Verification items for the finished model (mm, model axes). Give positions to 0.01 mm unless a question says otherwise; leave off trailing zeros. Order: outer loops, then holes, each group sorted by start corner. A loop starts at its lowest first (then second) coordinate and runs counter-clockwise, first axis right, second up.
from build123d import *

# Parameters (mm, degrees)
BOSS_EXTRUDE2_DEPTH     = 3
CUT_EXTRUDE1_DEPTH      = 330.393231219
CUT_EXTRUDE1_DEPTH_BACK = 3
SKETCH4_W               = 17.5
SKETCH4_H               = 12
CUT_EXTRUDE2_DEPTH      = 10
SKETCH5_R               = 5.7
CUT_EXTRUDE3_DEPTH      = 10
SKETCH6_R               = 6.5
CUT_EXTRUDE4_DEPTH      = 10
SKETCH7_R               = 1.5
CUT_EXTRUDE5_DEPTH      = 10


with BuildPart() as part:
    # Sketch1 → Boss-Extrude2 (new body)
    with BuildSketch(Plane(origin=(0, 0, 0), x_dir=(0, 0, -1), z_dir=(1, 0, 0))):
        Polygon((18.855403516, 70), (318.855403516, 70), (318.855403516, 55), (321.855403516, 55), (321.855403516, 15), (318.855403516, 15), (318.855403516, 0), (18.855403516, 0), (18.855403516, 15), (15.855403516, 15), (15.855403516, 55), (18.855403516, 55), align=None)
    extrude(amount=BOSS_EXTRUDE2_DEPTH)

    # Sketch3 → Cut-Extrude1 (cut, two sides: drawn at the far end of the back side and taken through both)
    with BuildSketch(Plane(origin=(3, 0, 0), x_dir=(0, 0, -1), z_dir=(1, 0, 0)).offset(-CUT_EXTRUDE1_DEPTH_BACK)):
        Polygon((48.855403516, 643.663019898), (48.855403516, 70), (48.855403516, 67), (288.855403516, 67), (288.855403516, 70), (288.855403516, 643.663019898), (288.855403516, 1790.989059693), (48.855403516, 1790.989059693), align=None)
    extrude(amount=CUT_EXTRUDE1_DEPTH + CUT_EXTRUDE1_DEPTH_BACK, mode=Mode.SUBTRACT)

    # Sketch4 → Cut-Extrude2 (cut)
    with BuildSketch(Plane(origin=(3, 0, 0), x_dir=(0, 0, -1), z_dir=(1, 0, 0))):
        with Locations((250.105403516, 31)):
            Rectangle(SKETCH4_W, SKETCH4_H)
    extrude(amount=-CUT_EXTRUDE2_DEPTH, mode=Mode.SUBTRACT)

    # Sketch5 → Cut-Extrude3 (cut)
    with BuildSketch(Plane(origin=(3, 0, 0), x_dir=(0, 0, -1), z_dir=(1, 0, 0))):
        with Locations((201.355403516, 30.5)):
            Circle(SKETCH5_R)
    extrude(amount=-CUT_EXTRUDE3_DEPTH, mode=Mode.SUBTRACT)

    # Sketch6 → Cut-Extrude4 (cut)
    with BuildSketch(Plane(origin=(3, 0, 0), x_dir=(0, 0, -1), z_dir=(1, 0, 0))):
        with Locations((92.990637001, 36.382151617)):
            Circle(SKETCH6_R)
    extrude(amount=-CUT_EXTRUDE4_DEPTH, mode=Mode.SUBTRACT)

    # Sketch7 → Cut-Extrude5 (cut)
    with BuildSketch(Plane(origin=(3, 0, 0), x_dir=(0, 0, -1), z_dir=(1, 0, 0))):
        with Locations((268.855403516, 3)):
            Circle(SKETCH7_R)
        with Locations((168.855403516, 3)):
            Circle(SKETCH7_R)
        with Locations((68.855403516, 3)):
            Circle(SKETCH7_R)
    extrude(amount=-CUT_EXTRUDE5_DEPTH, mode=Mode.SUBTRACT)


solid = part.part
(1) Release check for a two-part mould opening along Z. For faces 1 (the cylindrical face through (1.52, 28.32, -206.62)), 2 (the flat face through (3, 35, -171)) record: pulls with the +Z half, pulls with the -Z half, needs draft (parallel to the pull), parting line crosses it, or undercut.
Solved:
face 1: undercut
face 2: needs draft
(2) Section check B-B, the plane x = 1.5. Enter the section's corners in (y, z), then the cut area to 3 significant figures.
Solved:
outline: (0, -318.86) - (15, -318.86) - (15, -321.86) - (55, -321.86) - (55, -318.86) - (70, -318.86) - (70, -288.86) - (67, -288.86) - (67, -48.86) - (70, -48.86) - (70, -18.86) - (55, -18.86) - (55, -15.86) - (15, -15.86) - (15, -18.86) - (0, -18.86) - close; hole circle Ø3 at (3, -268.86); hole circle Ø3 at (3, -168.86); hole circle Ø3 at (3, -68.86); hole circle Ø11.4 at (30.5, -201.36); hole (25, -258.86) - (37, -258.86) - (37, -241.36) - (25, -241.36) - close; hole circle Ø13 at (36.38, -92.99)
area: 20,100 mm2
(3) Go/stop test with flat-tipped pins: pin 1 (1.5 mm diameter, centred on x = 2, z = -249, fed in from +Y); pin 2 (1.5 mm diameter, centred on x = 1, y = 5.5, fed in from -Z); pin 3 (1.5 mm diameter, centred on x = 2, y = 7, fed in from +Z). Record where each tip stops, or that it passes through.
Solved:
pin 1: stops at y = 67
pin 2: stops at z = -318.86
pin 3: stops at z = -18.86
(4) Scan lines: line 1 (Y direction, x = 1.1, z = -150.5); line 2 (Z direction, x = 2.25, y = 28); line 3 (Y direction, x = 0.4, z = -91). Record each from-to range of solid material in increasing order.
Solved:
line 1: y = 0 to 67
line 2: z = -321.86 to -258.86, -241.36 to -206.48, -196.23 to -15.86
line 3: y = 0 to 30.19, 42.57 to 67
(5) Section check C-C, the plane z = -108.5. Enter the section's corners in (x, y).
Solved:
outline: (0, 0) - (3, 0) - (3, 67) - (0, 67) - close
(6) Section check A-A, the plane z = -248. Enter the section's corners in (x, y).
Solved:
outline: (0, 0) - (3, 0) - (3, 25) - (0, 25) - close; (0, 37) - (3, 37) - (3, 67) - (0, 67) - close
